The drawing under review shows one solid part. Ordinate dimensions are in mm from its lowest x, y, z. A direction names the side the tool comes from. Round coordinates to 2 decimals unless told otherwise and drop trailing zeros. Order: outer loops, then holes, each group sorted by start corner. A loop starts at its lowest first (then second) coordinate and runs counter-clockwise, first axis right, second up. Notation, with made-up numbers: (-26, 42.5) -> (11, 42.5) arc R15 cw to (11, 47.5) -> close; hole circle Ø8 at (-39.5, 67). An arc over 180 degrees is marked (long way). Return JSON: item names as keys, results as strings. Group by question number.
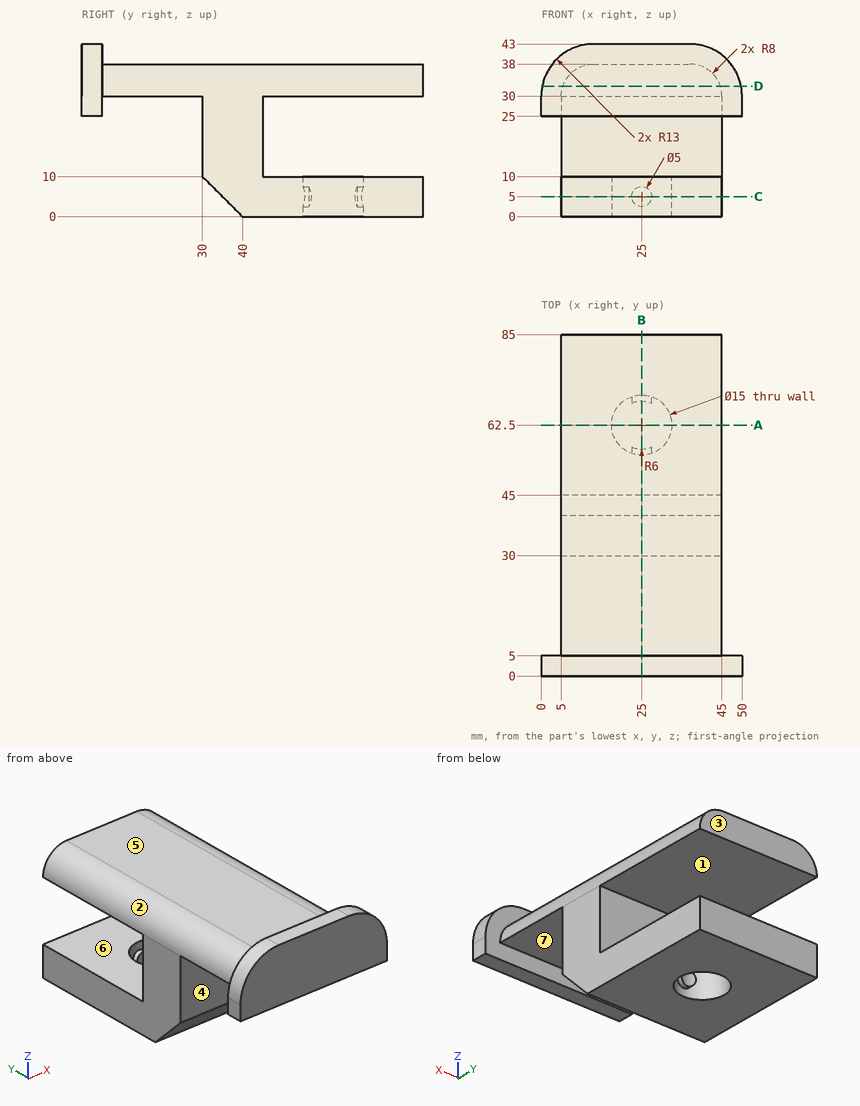
Item 1: For the marked faces 1, 2 and 3, list the 3-axis set-ups (+Z, -Z, +X, -X, +Y, -Y) from which the entire face can be reached by the end or side of a thin tool; tool diameter is ignored.
Item 2: Consider section D-D on z = 32.5. State the section outline as (x, y) points, plus the area to 3 significant figures.
Item 3: Consider section B-B on x = 25. State the section outline as (y, z) points, plus the area to 4 significant figures.
Item 4: Insertion check: pin 1 Ø6 at (x, y) = (11.5, 70.5) entering from +Z; pin 2 Ø2 at (x, z) = (10.5, 12.5) entering from +Y; pin 3 Ø5.5 at (x, y) = (21.5, 2) entering from -Z; pin 4 Ø9 at (y, z) = (51, 22.5) entering from -X. Each pin has a flat end and moves straight along its axis. Give the tip position at first contact, or say it passes through.
Item 5: The part is to be moulded in two halves that separate along Z. For the marked faces 4, 5, 6 and 7, say which applies: +Z half, -Z half, draft (parallel to the pull), parting line (faces both ways), or undercut.
Item 6: Consider section C-C on z = 5. State the section outline as (x, y) points, plus the area to 3 significant figures.
Item 7: Consider section A-A on y = 62.5. Give the number of separate pieces and of enclosed holes in the cut face, plus the area to 3 significant figures.
Item 8: Wall thickness on line 1 along Z through (x, y) = (15, 80.5); line 2 along X through (y, z) = (62, 5); line 3 along Y through (x, z) = (25, 3): over which ranges is each line inside the solid? List them lowest first.
Values:
{
 "1": {"face 1": "+X, -X, +Y", "face 2": "+Z, -X, +Y", "face 3": "+Z, -Z, +X, -X, +Y"},
 "2": {"outline": "(0.24, 0) -> (49.76, 0) -> (49.76, 5) -> (44.6, 5) -> (44.6, 85) -> (5.4, 85) -> (5.4, 5) -> (0.24, 5) -> close", "area": "3,380 mm^2"},
 "3": {"outline": "(0, 25) -> (5, 25) -> (5, 30) -> (30, 30) -> (30, 10) -> (40, 0) -> (55, 0) -> (55, 2.5) -> (56.5, 2.5) -> (56.5, 7.5) -> (55, 7.5) -> (55, 10) -> (45, 10) -> (45, 30) -> (85, 30) -> (85, 38) -> (5, 38) -> (5, 43) -> (0, 43) -> close; (68.5, 2.5) -> (70, 2.5) -> (70, 0) -> (85, 0) -> (85, 10) -> (70, 10) -> (70, 7.5) -> (68.5, 7.5) -> close", "area": "1,395 mm^2"},
 "4": {"pin 1": "z = 38", "pin 2": "y = 45", "pin 3": "z = 25", "pin 4": "through"},
 "5": {"face 4": "draft", "face 5": "+Z half", "face 6": "undercut", "face 7": "-Z half"},
 "6": {"outline": "(5, 35) -> (45, 35) -> (45, 85) -> (5, 85) -> close; hole (22.5, 55.43) -> (22.5, 57.05) arc R6 ccw to (27.5, 57.05) -> (27.5, 55.43) arc R7.5 ccw to (27.5, 69.57) -> (27.5, 67.95) arc R6 ccw to (22.5, 67.95) -> (22.5, 69.57) arc R7.5 ccw to start", "area": "1,840 mm^2"},
 "7": {"separate pieces": "3", "enclosed holes": "0", "area": "543 mm^2"},
 "8": {"line 1": "0 to 10, 30 to 38", "line 2": "5 to 17.52, 32.48 to 45", "line 3": "37 to 56.5, 68.5 to 85"}
}
